from build123d import *

# Parameters (mm, degrees)
SKETCH1_R           = 50
SKETCH1_R_2         = 5
BOSS_EXTRUDE1_DEPTH = 50
SKETCH2_R           = 37.5
SKETCH2_R_2         = 5
BOSS_EXTRUDE2_DEPTH = 8
SKETCH3_R           = 39
SKETCH3_R_2         = 5
BOSS_EXTRUDE3_DEPTH = 2
BOSS_EXTRUDE4_START = 10
SKETCH4_R           = 15
SKETCH4_R_2         = 5
BOSS_EXTRUDE4_DEPTH = 10


with BuildPart() as part:
    # Sketch1 → Boss-Extrude1 (new body)
    with BuildSketch(Plane.XY):
        Circle(SKETCH1_R)
        Circle(SKETCH1_R_2, mode=Mode.SUBTRACT)
    extrude(amount=BOSS_EXTRUDE1_DEPTH)

    # Sketch2 → Boss-Extrude2 (add)
    with BuildSketch(Plane.XY.offset(50)):
        Circle(SKETCH2_R)
        Circle(SKETCH2_R_2, mode=Mode.SUBTRACT)
    extrude(amount=BOSS_EXTRUDE2_DEPTH)

    # Sketch3 → Boss-Extrude3 (add)
    with BuildSketch(Plane.XY.offset(58)):
        Circle(SKETCH3_R)
        Circle(SKETCH3_R_2, mode=Mode.SUBTRACT)
    extrude(amount=BOSS_EXTRUDE3_DEPTH)

    # Sketch4 → Boss-Extrude4 (add)
    with BuildSketch(Plane(origin=(0, 0, 0), x_dir=(-1, 0, 0), z_dir=(0, 0, -1)).offset(BOSS_EXTRUDE4_START)):
        with Locations(Location((0, 0, 0), (0, 0, 180))):
            Circle(SKETCH4_R)
        Circle(SKETCH4_R_2, mode=Mode.SUBTRACT)
    extrude(amount=-BOSS_EXTRUDE4_DEPTH)


solid = part.part
Work out the finished part from the listing and answer in its coordinate system (mm). A direction names the side the tool comes from. Give positions to 0.01 mm unless a question says otherwise; leave off trailing zeros. Order: outer loops, then holes, each group sorted by start corner. A loop starts at its lowest first (then second) coordinate and runs counter-clockwise, first axis right, second up. Notation, with made-up numbers: (30.5, -36) -> (56.5, -36) arc R17 cw to (56.5, -4) -> close; hole circle Ø2 at (-20.75, 4.25). An arc over 180 degrees is marked (long way). Answer as a JSON object with one key per item and string values. Group by question number.
1. Section D-D on y = 34 is taken. Determine the outline of the cut face in (x, z), plus the area to 3 significant figures.
2. A tool of negligible diameter and unlimited length cuts with its end or side. For faces 5 (the flat face through (-4, -4, -10)), 6 (the cylindrical face through (-5.077, 38.668, 58.986)), from which of +Z, -Z, +X, -X, +Y, -Y can it reach the whole face along a straight path? Write none if from no direction.
3. Section C-C on z = 35 is taken. Determine the outline of the cut face in (x, y).
4. The mould has two halves that part along Z. Classify faces 1 (the cylindrical face through (-4.88, 37.18, 53.94)), 2 (the flat face through (-20, 32, 58)), 3 (the flat face through (-12, -10, 0)), 4 (the cylindrical face through (8.06, -12.65, -5.07)): released by +Z, released by -Z, zero draft, split by the parting line, or undercut.
5. Flat-ended cylindrical pins translate along their axes: pin 1 Ø3 at (y, z) = (-40, 13) entering from +X; pin 2 Ø10 at (y, z) = (-16.5, -1) entering from +X; pin 3 Ø8 at (x, y) = (12.5, 24.5) entering from -Z. Find the tip coordinate at first contact, or state that the pin passes through.
6. Consider line 1 along Y through (x, z) = (0, 35); line 2 along Z through (x, y) = (-26.5, -31); line 3 along Z through (x, y) = (-3.5, -37.5). Determine where each line is inside the solid, lowest interval first. Write a range as [from, to].
Result sheet:
{
 "1": {"outline": "(-36.66, 0) -> (36.66, 0) -> (36.66, 50) -> (15.82, 50) -> (15.82, 58) -> (19.1, 58) -> (19.1, 60) -> (-19.1, 60) -> (-19.1, 58) -> (-15.82, 58) -> (-15.82, 50) -> (-36.66, 50) -> close", "area": "4,000 mm^2"},
 "2": {"face 5": "-Z, +X, -X, +Y, -Y", "face 6": "+Z"},
 "3": {"outline": "circle Ø100 at (0, 0); hole circle Ø10 at (0, 0)"},
 "4": {"face 1": "undercut", "face 2": "undercut", "face 3": "released by -Z", "face 4": "zero draft"},
 "5": {"pin 1": "stops at x = 31.9", "pin 2": "stops at x = 48.64", "pin 3": "stops at z = 0"},
 "6": {"line 1": "y = [-50, -5], [5, 50]", "line 2": "z = [0, 50]", "line 3": "z = [0, 50], [58, 60]"}
}
